from build123d import *

# Parameters (mm, degrees)
SZKIC1_W                    = 358
SZKIC1_H                    = 451.5
DODANIE_WYCI_GNI_CIE1_DEPTH = 10
WYTNIJ_WYCI_GNI_CIE1_DEPTH  = 10
WYTNIJ_WYCI_GNI_CIE2_DEPTH  = 10
WYTNIJ_WYCI_GNI_CIE3_DEPTH  = 10
SZKIC8_W                    = 6.4
SZKIC8_H                    = 20.4
WYTNIJ_WYCI_GNI_CIE4_DEPTH  = 10
SZYK_LINIOWY1_COUNT         = 2
SZYK_LINIOWY1_PITCH         = 300
SZKIC9_R                    = 1.55
WYTNIJ_WYCI_GNI_CIE5_DEPTH  = 10
SZYK_LINIOWY2_COUNT         = 2
SZYK_LINIOWY2_PITCH         = 60
SZYK_LINIOWY2_COUNT_DIR2    = 2
SZYK_LINIOWY2_PITCH_DIR2    = 310
WYTNIJ_WYCI_GNI_CIE6_DEPTH  = 794.025959913
SZKIC12_R                   = 1.55
WYTNIJ_WYCI_GNI_CIE7_DEPTH  = 10
SZKIC15_R                   = 1.5
WYTNIJ_WYCI_GNI_CIE9_DEPTH  = 10
SZKIC17_R                   = 1.55
WYTNIJ_WYCI_GNI_CIE10_DEPTH = 10
SZKIC19_W                   = 20.4
SZKIC19_H                   = 6.4
SZKIC19_W_2                 = 30.4
WYTNIJ_WYCI_GNI_CIE11_DEPTH = 10
SZKIC23_R                   = 1.55
SZKIC23_W                   = 14.4
SZKIC23_H                   = 6.4
SZKIC23_W_2                 = 17.9
WYTNIJ_WYCI_GNI_CIE12_DEPTH = 10
SZKIC31_R                   = 1.55
WYTNIJ_WYCI_GNI_CIE15_DEPTH = 10
SZYK_LINIOWY3_COUNT         = 2
SZYK_LINIOWY3_PITCH         = 180
SZKIC33_W                   = 6.4
SZKIC33_H                   = 20.4
WYTNIJ_WYCI_GNI_CIE16_DEPTH = 10
SZYK_LINIOWY4_COUNT         = 3
SZYK_LINIOWY4_PITCH         = 60
SZKIC35_R                   = 1.55
SZKIC35_W                   = 20.9
SZKIC35_H                   = 6.4
SZKIC35_W_2                 = 14.4
WYTNIJ_WYCI_GNI_CIE17_DEPTH = 10
SZYK_LINIOWY5_COUNT         = 2
SZYK_LINIOWY5_PITCH         = 155
WYTNIJ_WYCI_GNI_CIE18_DEPTH = 10
SZKIC37_W                   = 12
SZKIC37_H                   = 20
WYTNIJ_WYCI_GNI_CIE19_DEPTH = 10
SZKIC39_R                   = 1.55
WYTNIJ_WYCI_GNI_CIE21_DEPTH = 10


with BuildPart() as part:
    # Szkic1 → Dodanie-wyciągnięcie1 (new body)
    with BuildSketch(Plane.XY):
        with Locations((-429.368459045, -282.853962956)):
            Rectangle(SZKIC1_W, SZKIC1_H)
    extrude(amount=DODANIE_WYCI_GNI_CIE1_DEPTH)

    # Szkic2 → Wytnij-wyciągnięcie1 (cut)
    with BuildSketch(Plane(origin=(0, 0, 0), x_dir=(-1, 0, 0), z_dir=(0, 0, -1))):
        Polygon((608.368459045, -387.603962956), (500.368459045, -57.103962956), (608.368459045, -57.103962956), align=None)
    extrude(amount=-WYTNIJ_WYCI_GNI_CIE1_DEPTH, mode=Mode.SUBTRACT)

    # Szkic3 → Wytnij-wyciągnięcie2 (cut)
    with BuildSketch(Plane.XY.offset(10)):
        with BuildLine():
            Line((-570.368459045, -508.603962956), (-290.368459045, -508.603962956))
            ThreePointArc((-290.368459045, -508.603962956), (-297.690789516, -490.926293426), (-315.368459045, -483.603962956))
            Line((-315.368459045, -483.603962956), (-545.368459045, -483.603962956))
            ThreePointArc((-545.368459045, -483.603962956), (-563.046128575, -490.926293426), (-570.368459045, -508.603962956))
        make_face()
    extrude(amount=-WYTNIJ_WYCI_GNI_CIE2_DEPTH, mode=Mode.SUBTRACT)

    # Szkic4 → Wytnij-wyciągnięcie3 (cut)
    with BuildSketch(Plane.XY.offset(10)):
        with BuildLine():
            Line((-491.890848015, -393.103962956), (-373.368459045, -393.103962956))
            ThreePointArc((-373.368459045, -393.103962956), (-345.084187798, -381.388234203), (-333.368459045, -353.103962956))
            Line((-333.368459045, -353.103962956), (-333.368459045, -217.103962956))
            ThreePointArc((-333.368459045, -217.103962956), (-345.084187798, -188.819691708), (-373.368459045, -177.103962956))
            Line((-373.368459045, -177.103962956), (-447.449093098, -177.103962956))
            ThreePointArc((-447.449093098, -177.103962956), (-470.93331873, -184.723549949), (-485.470539353, -204.679405632))
            Line((-485.470539353, -204.679405632), (-529.91229427, -340.679405632))
            ThreePointArc((-529.91229427, -340.679405632), (-524.271261022, -376.588188587), (-491.890848015, -393.103962956))
        make_face()
    extrude(amount=-WYTNIJ_WYCI_GNI_CIE3_DEPTH, mode=Mode.SUBTRACT)

    # Szkic8 → Wytnij-wyciągnięcie4 (cut)
    with BuildSketch(Plane.XY.offset(10)):
        with Locations((-259.368459045, -119.603962956)):
            Rectangle(SZKIC8_W, SZKIC8_H)
    wytnij_wyci_gni_cie4 = extrude(amount=-WYTNIJ_WYCI_GNI_CIE4_DEPTH, mode=Mode.SUBTRACT)

    # Szyk liniowy1: Wytnij-wyciągnięcie4 ×2
    with Locations(*[(0, -i * SZYK_LINIOWY1_PITCH, 0) for i in range(1, SZYK_LINIOWY1_COUNT)]):
        add(wytnij_wyci_gni_cie4, mode=Mode.SUBTRACT)

    # Szkic9 → Wytnij-wyciągnięcie5 (cut)
    with BuildSketch(Plane.XY.offset(10)):
        with Locations((-259.368459045, -89.603962956)):
            Circle(SZKIC9_R)
    wytnij_wyci_gni_cie5 = extrude(amount=-WYTNIJ_WYCI_GNI_CIE5_DEPTH, mode=Mode.SUBTRACT)

    # Szyk liniowy2: Wytnij-wyci_gni_cie5 2 × 2
    with Locations(*[Vector(0, -1, 0) * (i * SZYK_LINIOWY2_PITCH) + Vector(0, -1, 0) * (j * SZYK_LINIOWY2_PITCH_DIR2) for i in range(SZYK_LINIOWY2_COUNT) for j in range(SZYK_LINIOWY2_COUNT_DIR2) if (i, j) != (0, 0)]):
        add(wytnij_wyci_gni_cie5, mode=Mode.SUBTRACT)

    # Szkic10 → Wytnij-wyciągnięcie6 (cut, through all)
    with BuildSketch(Plane.XY.offset(10)):
        with BuildLine():
            Line((-256.368459045, -57.103962956), (-250.368459045, -57.103962956))
            Line((-250.368459045, -57.103962956), (-250.368459045, -63.103962956))
            ThreePointArc((-250.368459045, -63.103962956), (-252.125818358, -58.861322269), (-256.368459045, -57.103962956))
        make_face()
        with BuildLine():
            Line((-502.621218356, -63.997823625), (-500.368459045, -57.103962956))
            Line((-500.368459045, -57.103962956), (-493.115856793, -57.103962956))
            ThreePointArc((-493.115856793, -57.103962956), (-498.986913201, -59.008859704), (-502.621218356, -63.997823625))
        make_face()
    extrude(amount=-WYTNIJ_WYCI_GNI_CIE6_DEPTH, mode=Mode.SUBTRACT)

    # Szkic12 → Wytnij-wyciągnięcie7 (cut)
    with BuildSketch(Plane.XY.offset(10)):
        with Locations((-593.368459045, -397.873962956)):
            Circle(SZKIC12_R)
        with Locations((-593.368459045, -446.553962956)):
            Circle(SZKIC12_R)
        Polygon((-602.568459045, -406.123962956), (-602.568459045, -438.803962956), (-596.368459045, -438.803962956), (-590.168459045, -438.803962956), (-590.168459045, -406.123962956), (-596.368459045, -406.123962956), align=None)
    extrude(amount=-WYTNIJ_WYCI_GNI_CIE7_DEPTH, mode=Mode.SUBTRACT)

    # Szkic15 → Wytnij-wyciągnięcie9 (cut)
    with BuildSketch(Plane.XY.offset(10)):
        with Locations((-295.368459045, -471.603962956)):
            Circle(SZKIC15_R)
        with Locations((-323.368459045, -471.603962956)):
            Circle(SZKIC15_R)
        with Locations((-375.368459045, -471.603962956)):
            Circle(SZKIC15_R)
        with Locations((-427.368459045, -471.603962956)):
            Circle(SZKIC15_R)
        with Locations((-479.368459045, -471.603962956)):
            Circle(SZKIC15_R)
        with Locations((-531.368459045, -471.603962956)):
            Circle(SZKIC15_R)
        with Locations((-583.368459045, -471.603962956)):
            Circle(SZKIC15_R)
        with Locations((-338.368459045, -449.412668339)):
            Circle(SZKIC15_R)
    extrude(amount=-WYTNIJ_WYCI_GNI_CIE9_DEPTH, mode=Mode.SUBTRACT)

    # Szkic17 → Wytnij-wyciągnięcie10 (cut)
    with BuildSketch(Plane.XY.offset(10)):
        with Locations((-300.868459045, -82.814883616)):
            Circle(SZKIC17_R)
        with Locations((-310.868459045, -82.814883616)):
            Circle(SZKIC17_R)
        with Locations((-300.868459045, -137.814883616)):
            Circle(SZKIC17_R)
        with Locations((-310.868459045, -137.814883616)):
            Circle(SZKIC17_R)
        Polygon((-305.868459045, -95.403962953), (-316.068459045, -95.403962953), (-316.068459045, -125.803962953), (-305.868459045, -125.803962953), (-295.668459045, -125.803962953), (-295.668459045, -95.403962953), align=None)
    wytnij_wyci_gni_cie10 = extrude(amount=-WYTNIJ_WYCI_GNI_CIE10_DEPTH, mode=Mode.SUBTRACT)

    # Szkic19 → Wytnij-wyciągnięcie11 (cut)
    with BuildSketch(Plane.XY.offset(10)):
        with Locations((-305.868459045, -66.103962956)):
            Rectangle(SZKIC19_W, SZKIC19_H)
        with Locations((-383.368459045, -66.103962956)):
            Rectangle(SZKIC19_W_2, SZKIC19_H)
        with Locations((-460.868459045, -66.103962956)):
            Rectangle(SZKIC19_W, SZKIC19_H)
    extrude(amount=-WYTNIJ_WYCI_GNI_CIE11_DEPTH, mode=Mode.SUBTRACT)

    # Szkic23 → Wytnij-wyciągnięcie12 (cut)
    with BuildSketch(Plane.XY.offset(10)):
        with Locations((-322.868459045, -420.103962956)):
            Circle(SZKIC23_R)
        with Locations((-279.368459045, -420.103962956)):
            Rectangle(SZKIC23_W, SZKIC23_H)
        with Locations((-310.118459045, -420.103962956)):
            Rectangle(SZKIC23_W_2, SZKIC23_H)
    extrude(amount=-WYTNIJ_WYCI_GNI_CIE12_DEPTH, mode=Mode.SUBTRACT)

    # Szkic31 → Wytnij-wyciągnięcie15 (cut)
    with BuildSketch(Plane(origin=(0, 0, 0), x_dir=(-1, 0, 0), z_dir=(0, 0, -1))):
        with Locations((324.868459045, -377.603962956)):
            Circle(SZKIC31_R)
    wytnij_wyci_gni_cie15 = extrude(amount=-WYTNIJ_WYCI_GNI_CIE15_DEPTH, mode=Mode.SUBTRACT)

    # Szyk liniowy3: Wytnij-wyciągnięcie15 ×2
    with Locations(*[(0, i * SZYK_LINIOWY3_PITCH, 0) for i in range(1, SZYK_LINIOWY3_COUNT)]):
        add(wytnij_wyci_gni_cie15, mode=Mode.SUBTRACT)

    # Szkic33 → Wytnij-wyciągnięcie16 (cut)
    with BuildSketch(Plane(origin=(0, 0, 0), x_dir=(-1, 0, 0), z_dir=(0, 0, -1))):
        with Locations((324.868459045, -347.603962956)):
            Rectangle(SZKIC33_W, SZKIC33_H)
    wytnij_wyci_gni_cie16 = extrude(amount=-WYTNIJ_WYCI_GNI_CIE16_DEPTH, mode=Mode.SUBTRACT)

    # Szyk liniowy4: Wytnij-wyciągnięcie16 ×3
    with Locations(*[(0, i * SZYK_LINIOWY4_PITCH, 0) for i in range(1, SZYK_LINIOWY4_COUNT)]):
        add(wytnij_wyci_gni_cie16, mode=Mode.SUBTRACT)

    # Szkic35 → Wytnij-wyciągnięcie17 (cut)
    with BuildSketch(Plane(origin=(0, 0, 0), x_dir=(-1, 0, 0), z_dir=(0, 0, -1))):
        with Locations((293.818459045, -394.603962956)):
            Circle(SZKIC35_R)
        with Locations((311.618459045, -394.603962956)):
            Rectangle(SZKIC35_W, SZKIC35_H)
        with Locations((279.368459045, -394.603962956)):
            Rectangle(SZKIC35_W_2, SZKIC35_H)
    extrude(amount=-WYTNIJ_WYCI_GNI_CIE17_DEPTH, mode=Mode.SUBTRACT)

    # Szyk liniowy5: Wytnij-wyciągnięcie10 ×2
    with Locations(*[(-i * SZYK_LINIOWY5_PITCH, 0, 0) for i in range(1, SZYK_LINIOWY5_COUNT)]):
        add(wytnij_wyci_gni_cie10, mode=Mode.SUBTRACT)

    # Szkic36 → Wytnij-wyciągnięcie18 (cut)
    with BuildSketch(Plane(origin=(0, 0, 0), x_dir=(-1, 0, 0), z_dir=(0, 0, -1))):
        with BuildLine():
            Line((607.873820609, -386.090277741), (608.368459045, -387.603962956))
            Line((608.368459045, -387.603962956), (608.368459045, -389.196417072))
            ThreePointArc((608.368459045, -389.196417072), (608.244025248, -387.623778467), (607.873820609, -386.090277741))
        make_face()
    extrude(amount=-WYTNIJ_WYCI_GNI_CIE18_DEPTH, mode=Mode.SUBTRACT)

    # Szkic37 → Wytnij-wyciągnięcie19 (cut)
    with BuildSketch(Plane(origin=(0, 0, 0), x_dir=(-1, 0, 0), z_dir=(0, 0, -1))):
        with Locations((309.868459045, -279.603962956)):
            Rectangle(SZKIC37_W, SZKIC37_H)
    extrude(amount=-WYTNIJ_WYCI_GNI_CIE19_DEPTH, mode=Mode.SUBTRACT)

    # Szkic39 → Wytnij-wyciągnięcie21 (cut)
    with BuildSketch(Plane(origin=(0, 0, 0), x_dir=(-1, 0, 0), z_dir=(0, 0, -1))):
        with Locations((271.368459045, -190.053962956)):
            Circle(SZKIC39_R)
        with Locations((271.368459045, -173.153962956)):
            Circle(SZKIC39_R)
    extrude(amount=-WYTNIJ_WYCI_GNI_CIE21_DEPTH, mode=Mode.SUBTRACT)


solid = part.part
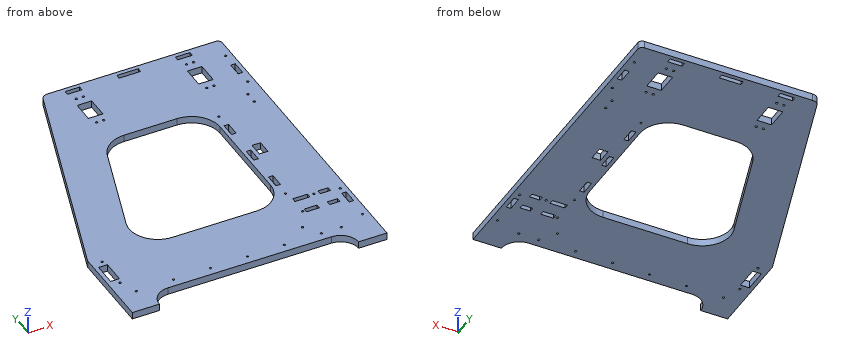
Here's how the part is built. I have some questions about the finished solid (model axes, mm). Round coordinates to 2 decimals unless told otherwise and drop trailing zeros. Loops run counter-clockwise (first coordinate to the right, second up) from the corner with the lowest first, then second, coordinate; pieces in that order, holes last. Notation, with made-up numbers: M 83,7 L 115,7 A30 ccw 115,41 Z; hole C 76,85 d9. An arc over 180 degrees is marked long. Write each question's results on one line, items separated by ' | '. Start each with the question number.
(1) I want a section at A-A (y = -309). Please give me the cut outline in (x, z), then the cut area to 3 significant figures.
(2) Will these pins go through, and if not, where does the flat tip stop? P1, Ø2, axis at x = -431.5, z = 4, coming from the -Y side; P2, Ø3, axis at y = -106, z = 2.5, coming from the -X side.
(3) I want a section at B-B (z = 7.25). State how many separate pieces and enclosed holes the cut face has, then the cut area to 3 significant figures.
(4) If I drill on probe 1 along Y at (x, z) = (-274, 6); probe 2 along Y at (x, z) = (-271, 6); probe 3 along X at (y, z) = (-197, 4), over which ranges is the centre line in solid material (lowest first)? Write a range as from..to.
(5) I want a section at C-C (x = -539). Please give me the cut outline in (y, z).
Solved:
1) outline: M -582.68,0 L -519.56,0 L -519.56,10 L -582.68,10 Z; M -333.37,0 L -250.37,0 L -250.37,10 L -333.37,10 Z | area: 1,460 mm²
2) P1: stops at y = -483.6 | P2: stops at x = -516.84
3) separate pieces: 1 | enclosed holes: 45 | area: 96,400 mm²
4) probe 1: y = -508.6..-423.3, -416.9..-397.8, -391.4..-57.1 | probe 2: y = -508.6..-191.56, -188.55..-174.66, -171.65..-57.1 | probe 3: x = -546.08..-482.03, -338.79..-326.3, -323.44..-250.37
5) outline: M -483.6,0 L -175.32,0 L -175.32,10 L -483.6,10 Z
